from build123d import *

# Parameters (mm, degrees)
SKETCH004_W   = 250
SKETCH004_H   = 350
SKETCH004_W_2 = 72.514309
SKETCH004_H_2 = 79.45462
SKETCH004_W_3 = 72.51431
SKETCH004_W_4 = 93.749451
SKETCH004_H_3 = 80.706021
PAD004_DEPTH  = 12.7
POCKET_DEPTH  = 5


with BuildPart() as obj1:
    # Sketch004 → Pad004 (new body)
    with BuildSketch(Plane.XY):
        with Locations((749.003465, 175)):
            Rectangle(SKETCH004_W, SKETCH004_H)
        with Locations((695.260619, 285.27269)):
            Rectangle(SKETCH004_W_2, SKETCH004_H_2, mode=Mode.SUBTRACT)
        with Locations((802.74631, 285.27269)):
            Rectangle(SKETCH004_W_3, SKETCH004_H_2, mode=Mode.SUBTRACT)
        with Locations((749.232575, 86.171351)):
            Rectangle(SKETCH004_W_4, SKETCH004_H_3, mode=Mode.SUBTRACT)
    extrude(amount=PAD004_DEPTH)

    # Sketch005 (on Face18 of Pad004) → Pocket (cut)
    with BuildSketch(Plane.XY.offset(12.7)):
        Polygon((609.961363, 176), (861.003465, 176), (861.003465, 350), (874.003465, 350), (874.003465, 0), (614.691284, 0), (614.691284, 13), (861.003465, 13), (861.003465, 163), (609.961363, 163), align=None)
    extrude(amount=-POCKET_DEPTH, mode=Mode.SUBTRACT)


with BuildPart() as obj2:
    # Mirror: instance of obj1
    add(obj1.part.mirror(Plane(origin=(879.241577, 357.188568, 0), x_dir=(0, 1, 0), z_dir=(-1, 0, 0))))


solid = obj2.part
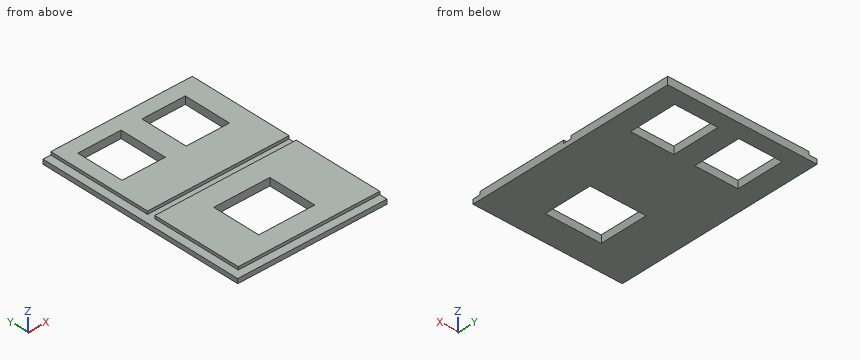
For this review, take the finished solid that the model builds, in its own axes (mm). Round coordinates to 2 decimals unless told otherwise and drop trailing zeros. Loops run counter-clockwise (first coordinate to the right, second up) from the corner with the lowest first, then second, coordinate; pieces in that order, holes last. Notation, with made-up numbers: (-10.75, -25) - (48.25, -25) arc R29 cw to (48.25, 4) - close; hole circle Ø10 at (12.5, 42.5). An arc over 180 degrees is marked (long way). Answer as CSV lines item,"result".
(1) Consider section A-A on z = 3.5. Give the boundary of the cut face in (x, y).
Checked values:
outline,"(884.48, 0) - (1134.48, 0) - (1134.48, 350) - (884.48, 350) - close; hole (919.48, 245.55) - (991.99, 245.55) - (991.99, 325) - (919.48, 325) - close; hole (962.38, 45.82) - (1056.13, 45.82) - (1056.13, 126.52) - (962.38, 126.52) - close; hole (1026.97, 245.55) - (1099.48, 245.55) - (1099.48, 325) - (1026.97, 325) - close"
(2) Consider section D-D on y = 67. Give the boundary of the cut face in (x, z).
Checked values:
outline,"(884.48, 0) - (962.38, 0) - (962.38, 12.7) - (897.48, 12.7) - (897.48, 7.7) - (884.48, 7.7) - close; (1056.13, 0) - (1134.48, 0) - (1134.48, 12.7) - (1056.13, 12.7) - close"
(3) Insertion check: P1, Ø2.5, axis at x = 1069, z = 9.5, coming from the -Y side; P2, Ø5.5, axis at y = 71.5, z = 11, coming from the -X side. Each pin has a flat end and moves straight along its axis. Give the tip position at first contact, or say it passes through.
Checked values:
P1,"stops at y = 13"
P2,"stops at x = 897.48"
(4) Wall thickness on line 1 (Y direction, x = 923, z = 12); line 2 (X direction, y = 271, z = 10.5); line 3 (Y direction, x = 969.5, z = 10.5): over which ranges is each line inside the solid? List them lowest first.
Checked values:
line 1,"y = 13 to 163, 176 to 245.55, 325 to 350"
line 2,"x = 897.48 to 919.48, 991.99 to 1026.97, 1099.48 to 1134.48"
line 3,"y = 13 to 45.82, 126.52 to 163, 176 to 245.55, 325 to 350"
(5) Consider section C-C on x = 927. Give the boundary of the cut face in (y, z), then the cut area to 3 significant figures.
Checked values:
outline,"(0, 0) - (245.55, 0) - (245.55, 12.7) - (176, 12.7) - (176, 7.7) - (163, 7.7) - (163, 12.7) - (13, 12.7) - (13, 7.7) - (0, 7.7) - close; (325, 0) - (350, 0) - (350, 12.7) - (325, 12.7) - close"
area,"3,310 mm2"
(6) Consider section B-B on y = 276. Give the boundary of the cut face in (x, z).
Checked values:
outline,"(884.48, 0) - (919.48, 0) - (919.48, 12.7) - (897.48, 12.7) - (897.48, 7.7) - (884.48, 7.7) - close; (991.99, 0) - (1026.97, 0) - (1026.97, 12.7) - (991.99, 12.7) - close; (1099.48, 0) - (1134.48, 0) - (1134.48, 12.7) - (1099.48, 12.7) - close"
